The listing builds one solid part. Answer for the finished solid, in the listing's coordinates (mm). A direction names the side the tool comes from. Give positions to 0.01 mm unless a question says otherwise; leave off trailing zeros. Write each loop counter-clockwise with the first axis right and the second up, starting at its lowest first coordinate (ties: lowest second). Pieces come first, ordered by that corner, then holes. Notation, with made-up numbers: M 14,-14 L 60,-14 A17 cw 60,7 Z; hole C 44,-6 d8. An arc over 180 degrees is marked long. Return JSON: item names as keys, results as strings.
from build123d import *
from build123d.topology import SkipClean

# Parameters (mm, degrees)
BOSS_EXTRUDE1_DEPTH      = 41
BOSS_EXTRUDE1_DEPTH_BACK = 18
SKETCH2_R                = 8.000000000000004
SKETCH3_R                = 9.5
BOSS_EXTRUDE2_DEPTH      = 28.5
BOSS_EXTRUDE3_DEPTH      = 5
BOSS_EXTRUDE4_DEPTH      = 25.451834
M3_5_TAPPED_HOLE1_D      = 2.9
FILLET2_R                = 2
SKETCH14_R               = 8.000000000000004
BOSS_EXTRUDE5_DEPTH      = 2
FILLET10_R               = 1
FILLET10_OF_MIRROR2_R    = 1
FILLET11_R               = 1
FILLET12_R               = 2
SKETCH15_W               = 47.04564696040835
SKETCH15_H               = 19.155839546122916
CUT_EXTRUDE2_DEPTH       = 123.75548779255048
SKETCH16_W               = 50.32184914639417
SKETCH16_H               = 9.010919354068848
CUT_EXTRUDE3_DEPTH       = 123.68683594132897


# Some blends are built 0.0001 mm under size
with BuildPart() as part:
    # Sketch2 → Boss-Extrude1 (new, two sides: drawn at the far end of the back side and taken through both)
    with BuildSketch(Plane.XY.offset(-BOSS_EXTRUDE1_DEPTH_BACK)):
        with BuildLine():
            Line((-12.5, -12.500000000000002), (12.5, -12.500000000000002))
            Line((12.5, -12.500000000000002), (12.5, 5.999999999999994))
            Line((12.5, 5.999999999999994), (12.5, 12.951833846988604))
            ThreePointArc((12.5, 12.951833846988604), (9.463639319119588, 15.311418315675832), (5.995365002334926, 16.97220075561143))
            Line((5.995365002334926, 16.97220075561143), (-1.0000000000000027, 16.97220075561143))
            Line((-1.0000000000000027, 16.97220075561143), (-5.995365002334937, 16.972200755611425))
            ThreePointArc((-5.995365002334937, 16.972200755611425), (-9.463639319119597, 15.311418315675827), (-12.5, 12.951833846988608))
            Line((-12.5, 12.951833846988608), (-12.5, 6.000000000000001))
            Line((-12.5, 6.000000000000001), (-12.5, -12.500000000000002))
        make_face()
        Circle(SKETCH2_R, mode=Mode.SUBTRACT)
    extrude(amount=BOSS_EXTRUDE1_DEPTH + BOSS_EXTRUDE1_DEPTH_BACK)

    # Sketch3 → Boss-Extrude2 (add)
    with BuildSketch(Plane.XY.offset(41)):
        with BuildLine():
            Line((-1.0000000000000016, 17.97498435543818), (0.727272727272726, 17.97498435543818))
            Line((0.727272727272726, 17.97498435543818), (8.769260939312526, 17.974984355438174))
            ThreePointArc((8.769260939312526, 17.974984355438174), (11.304195151298408, 16.498944571740374), (13.595959595959597, 14.667988364633844))
            Line((13.595959595959597, 14.667988364633844), (13.595959595959597, 6.224872228225638))
            Line((13.595959595959597, 6.224872228225638), (13.595959595959597, -12.5))
            Line((13.595959595959597, -12.5), (-13.500000000000002, -12.500000000000004))
            Line((-13.500000000000002, -12.500000000000004), (-13.500000000000002, 6.223411383455548))
            Line((-13.500000000000002, 6.223411383455548), (-13.500000000000002, 14.756354563373698))
            ThreePointArc((-13.500000000000002, 14.756354563373698), (-11.250328445445001, 16.535722236104803), (-8.769260939312526, 17.97498435543818))
            Line((-8.769260939312526, 17.97498435543818), (-1.0000000000000016, 17.97498435543818))
        make_face()
        with Locations(Location((-1.73e-15, 0, 0), (0, 0, 180))):
            Circle(SKETCH3_R, mode=Mode.SUBTRACT)
    boss_extrude2 = extrude(amount=BOSS_EXTRUDE2_DEPTH)

    # Mirror1: Boss-Extrude2 across plane
    add(boss_extrude2.mirror(Plane.XY.offset(11.5)))

    # Sketch4 → Boss-Extrude3 (add)
    with BuildSketch(Plane.XZ.offset(12.500000000000002)):
        Polygon((-13.500000000000002, 41), (-13.500000000000002, 69.5), (-18.500000000000004, 69.5), (-18.500000000000004, 42.75), (-18.500000000000004, 36.00000000000001), (-17.5, 36.00000000000001), (-17.5, -13), (-18.500000000000004, -13.000000000000002), (-18.500000000000004, -46.5), (-13.500000000000002, -46.5), (-13.500000000000002, -18.000000000000004), (-12.499999999999998, -18.000000000000004), (-12.5, 41), align=None)
        Polygon((18.595959595959595, 69.5), (13.595959595959597, 69.5), (13.595959595959597, 41), (12.5, 41), (12.5, -18.000000000000004), (13.595959595959597, -18.000000000000004), (13.595959595959597, -46.5), (18.5959595959596, -46.5), (18.595959595959595, -13), (17.5, -13.000000000000002), (17.5, 36.00000000000001), (18.595959595959595, 36.00000000000001), (18.595959595959595, 42.75), align=None)
        Polygon((13.595959595959597, -18.000000000000004), (12.5, -18.000000000000004), (12.5, 41), (13.595959595959597, 41), (13.595959595959597, 69.5), (-13.500000000000002, 69.5), (-13.500000000000002, 41), (-12.5, 41), (-12.499999999999998, -18.000000000000004), (-13.500000000000002, -18.000000000000004), (-13.500000000000002, -46.5), (13.595959595959597, -46.5), align=None)
    extrude(amount=BOSS_EXTRUDE3_DEPTH)

    # Sketch5 → Boss-Extrude4 (add)
    with BuildSketch(Plane(origin=(0, -12.500000000000002, 0), x_dir=(1, 0, 0), z_dir=(0, 1, 0))):
        Polygon((13.595959595959597, -41), (13.595959595959597, -69.5), (18.595959595959595, -69.5), (18.595959595959595, -36.00000000000001), (17.5, -36.00000000000001), (17.5, 13.000000000000002), (18.595959595959595, 13.000000000000002), (18.595959595959595, 46.5), (13.595959595959597, 46.5), (13.595959595959597, 18.000000000000004), (12.5, 18.000000000000004), (12.5, -41), align=None)
        Polygon((-18.500000000000004, -69.5), (-13.500000000000002, -69.5), (-13.500000000000002, -41), (-12.5, -41), (-12.499999999999998, 18.000000000000004), (-13.500000000000002, 18.000000000000004), (-13.500000000000002, 46.5), (-18.5, 46.5), (-18.500000000000004, 13.000000000000002), (-17.5, 13.000000000000002), (-17.5, -36.00000000000001), (-18.500000000000004, -36.00000000000001), align=None)
    extrude(amount=BOSS_EXTRUDE4_DEPTH)

    # M3.5 Tapped Hole1 (through all)
    with Locations(Plane(origin=(-1.179e-14, 16.97220075561143, 0), x_dir=(1, 6.9e-16, 0), z_dir=(-6.9e-16, 1, 0))):
        with Locations((-12.5, 15), (12.5, 15), (12.5, 35), (-12.5, 35)):
            m3_5_tapped_hole1 = Hole(M3_5_TAPPED_HOLE1_D / 2)

    # Fillet2
    fillet2_edges = [part.edges().sort_by_distance(p)[0] for p in [
        (18.595959595959595, 12.951834, -29.75),
        (-18.5, 12.951834, -29.75),
    ]]
    fillet(fillet2_edges, radius=FILLET2_R - 0.0001)  # a hair under: the kernel refuses the full size

    # Sketch14 → Boss-Extrude5 (add)
    with SkipClean():  # the faces are left unmerged after this step: merging them gives an invalid solid
        with BuildSketch(Plane.XY.offset(69.5)):
            with BuildLine():
                Line((13.595959595959597, 12.951833846988603), (-13.500000000000002, 12.951833846988603))
                Line((-13.500000000000002, 12.951833846988603), (-16.5, 12.951833846988603))
                ThreePointArc((-16.5, 12.951833846988604), (-17.914213562373096, 12.366047409361698), (-18.5, 10.951833846988603))
                Line((-18.500000000000004, 10.951833846988603), (-18.500000000000004, -17.5))
                Line((-18.500000000000004, -17.5), (18.595959595959595, -17.5))
                Line((18.595959595959595, -17.5), (18.595959595959595, 10.951833846988603))
                ThreePointArc((18.595959595959595, 10.951833846988603), (18.01017315833269, 12.366047409361698), (16.595959595959595, 12.951833846988603))
                Line((16.595959595959595, 12.951833846988604), (13.595959595959597, 12.951833846988603))
            make_face()
            Circle(SKETCH14_R, mode=Mode.SUBTRACT)
        boss_extrude5 = extrude(amount=BOSS_EXTRUDE5_DEPTH)

    # Fillet10
    fillet10_edges = [part.edges().sort_by_distance(p)[0] for p in [
        (0.04797979797979934, 12.951833846988603, 71.5),
        (-8.000000000000004, 9.8e-16, 71.5),
        (-17.914213562373096, 12.366047409361698, 71.5),
        (-18.500000000000004, -3.2740830765056987, 71.5),
        (0.04797979797979579, -17.5, 71.5),
        (18.595959595959595, -3.2740830765056987, 71.5),
        (18.01017315833269, 12.366047409361698, 71.5),
    ]]
    fillet(fillet10_edges, radius=FILLET10_R)

    # Mirror2: Boss-Extrude5 across plane
    with SkipClean():  # the faces are left unmerged after this step: merging them gives an invalid solid
        add(boss_extrude5.mirror(Plane.XY.offset(11.5)))

    # Fillet10 of Mirror2
    fillet10_of_mirror2_edges = [part.edges().sort_by_distance(p)[0] for p in [
        (0.04797979797979934, 12.951833846988603, -48.5),
        (-8.000000000000004, 9.8e-16, -48.5),
        (-17.914213562373096, 12.366047409361698, -48.5),
        (-18.500000000000004, -3.2740830765056987, -48.5),
        (0.04797979797979579, -17.5, -48.5),
        (18.595959595959595, -3.2740830765056987, -48.5),
        (18.01017315833269, 12.366047409361698, -48.5),
    ]]
    fillet(fillet10_of_mirror2_edges, radius=FILLET10_OF_MIRROR2_R)

    # Fillet11
    fillet11_edges = [part.edges().sort_by_distance(p)[0] for p in [
        (11.304195151298412, 16.498944571740378, 69.5),
        (1.78e-15, 17.974984355438178, 69.5),
        (-11.250328445445, 16.535722236104803, 69.5),
        (-11.250328445445, 16.535722236104803, -46.5),
        (1.78e-15, 17.974984355438178, -46.5),
        (11.304195151298412, 16.498944571740378, -46.5),
    ]]
    fillet(fillet11_edges, radius=FILLET11_R)

    # Fillet12
    # the kernel refuses this fillet: 2 mm, written as the material it adds along each edge
    with BuildSketch(Plane(origin=(-1.73e-15, 0, 41), x_dir=(-1, 1.2e-16, 0), z_dir=(1.2e-16, 1, 0))) as fillet12_piece_1:
        with BuildLine():
            CenterArc((7.5, 1.9364916731037098), FILLET12_R, 284.47751218593, 75.52248781407002)
            Line((8.000000000000004, 0), (8.010000000000003, -0.03872983346207093))
            ThreePointArc((8.010000000000003, -0.03872983346207093), (8.750000000000002, -0.03999999999999915), (9.5, -0.03999999999999915))
            Line((9.5, -0.03999999999999915), (9.54, 0))
            Line((9.54, 0), (9.54, 1.9364916731037098))
            Line((9.54, 1.9364916731037098), (9.5, 1.9364916731037098))
        make_face()
    revolve(axis=Axis((-1.73e-15, 0, 41), (0, 0, 1)))
    # the kernel refuses this fillet: 2 mm, written as the material it takes off along each edge
    with BuildSketch(Plane(origin=(-1.73e-15, 0, -18), x_dir=(1, 0, 0), z_dir=(0, -1, 0))) as fillet12_2_piece_1:
        with BuildLine():
            CenterArc((10.000000000000004, 1.9364916731037063), FILLET12_R, 180, 75.52248781406996)
            Line((8.000000000000004, 1.9364916731037063), (7.9600000000000035, 1.9364916731037063))
            Line((7.9600000000000035, 1.9364916731037063), (7.9600000000000035, 0))
            Line((7.9600000000000035, 0), (8.000000000000004, -0.03999999999999915))
            ThreePointArc((8.000000000000004, -0.03999999999999915), (8.750000000000002, -0.03999999999999915), (9.49, -0.03872983346207448))
            Line((9.49, -0.03872983346207448), (9.5, 0))
        make_face()
    revolve(axis=Axis((-1.73e-15, 0, -18), (0, 0, 1)), mode=Mode.SUBTRACT)

    # Mirror3: M3.5 Tapped Hole1 across plane
    with SkipClean():  # the faces are left unmerged after this step: merging them gives an invalid solid
        add(m3_5_tapped_hole1.mirror(Plane.XY.offset(11.5)), mode=Mode.SUBTRACT)

    # Sketch15 → Cut-Extrude2 (cut, through all)
    with BuildSketch(Plane.XY.offset(71.50000000000001)):
        with Locations((2.6415149640881275, 9.577919773061458)):
            Rectangle(SKETCH15_W, SKETCH15_H)
    extrude(amount=-CUT_EXTRUDE2_DEPTH, mode=Mode.SUBTRACT)

    # Sketch16 → Cut-Extrude3 (cut, through all)
    with BuildSketch(Plane(origin=(0, 0, -48.50000000000001), x_dir=(-1, 0, 0), z_dir=(0, 0, -1))):
        with Locations((0.38733031574332877, -17.005459677034427)):
            Rectangle(SKETCH16_W, SKETCH16_H)
    extrude(amount=-CUT_EXTRUDE3_DEPTH, mode=Mode.SUBTRACT)


solid = part.part
Item 1: Which of the six approach directions +Z, -Z, +X, -X, +Y, -Y give full straight-line access (tool end or side, diameter ignored) to faces 1 (the cylindrical face through (12.814, -6.337, -33.584)), 2 (the flat face through (-17.5, -6, 12)), 3 (the flat face through (-1.5, -8.2, 69.5))?
Geometry results:
{"face 1": "+Y, -Y", "face 2": "-X, +Y, -Y", "face 3": "+Y"}
Item 2: Determine the mould class of faces 4 (the cylindrical face through (0, -8, 70)), 5 (the flat face through (17.5, -6, 12)), 6 (the flat face through (0, -10, -48.5)), 7 (the flat face through (-18.5, -6, -30)) for opening direction X: +X half, -X half, draft (parallel to the pull), parting line (faces both ways), or undercut.
Geometry results:
{"face 4": "undercut", "face 5": "+X half", "face 6": "draft", "face 7": "-X half"}
Item 3: Given pin 1 Ø4.5 at (x, z) = (-12.5, 38) entering from +Y; pin 2 Ø3 at (x, y) = (4.5, -5) entering from +Z; pin 3 Ø4 at (y, z) = (-8, 11.5) entering from +X; pin 4 Ø1.2 at (x, y) = (18.5, -3.5) entering from +Z, each flat-ended and moving along its own axis, determine where each tip first touches the part or whether it passes through.
Geometry results:
{"pin 1": "stops at y = 0", "pin 2": "stops at z = 71.13", "pin 3": "stops at x = 17.5", "pin 4": "stops at z = 71.45"}
Item 4: A cutting plane is placed at D-D, the plane y = -2. Count the separate pieces of the cut face and the enclosed holes in it, plus the area to 3 significant figures.
Geometry results:
{"separate pieces": "2", "enclosed holes": "8", "area": "2,260 mm2"}
Item 5: A cutting plane is placed at B-B, the plane z = 58. Write down the section's boundary in (x, y), plus the area to 3 significant figures.
Geometry results:
{"outline": "M -18.5,-12.5 L -13.95,-12.5 L -13.95,0 L -18.5,0 Z; M -11.05,-12.5 L 11.05,-12.5 L 11.05,0 L 9.5,0 A9.5 cw -9.5,0 L -11.05,0 Z; M 13.95,-12.5 L 18.6,-12.5 L 18.6,0 L 13.95,0 Z", "area": "249 mm2"}
Item 6: A cutting plane is placed at A-A, the plane x = 12.5. Write down the section's boundary in (y, z), plus the area to 4 significant figures.
Geometry results:
{"outline": "M -12.5,-48.5 L 0,-48.5 L 0,-36.45 L -12.5,-36.45 Z; M -12.5,-33.55 L 0,-33.55 L 0,-16.45 L -12.5,-16.45 Z; M -12.5,-13.55 L 0,-13.55 L 0,36.55 L -12.5,36.55 Z; M -12.5,39.45 L 0,39.45 L 0,56.55 L -12.5,56.55 Z; M -12.5,59.45 L 0,59.45 L 0,71.5 L -12.5,71.5 Z", "area": "1,355 mm2"}
Item 7: Find the intervals of material crossed by line 1 (Z direction, x = -12.5, y = -8); line 2 (X direction, y = -9, z = 38); line 3 (X direction, y = -10.25, z = -36), in increasing order.
Geometry results:
{"line 1": "z = -48.5 to -36.45, -33.55 to -16.45, -13.55 to 36.55, 39.45 to 56.55, 59.45 to 71.5", "line 2": "x = -18.5 to -13.95, -11.05 to 11.05, 13.95 to 18.6", "line 3": "x = -18.5 to -13.55, -11.45 to 11.45, 13.55 to 18.6"}
Item 8: A cutting plane is placed at C-C, the plane z = -23. Write down the section's boundary in (x, y), plus the area to 3 significant figures.
Geometry results:
{"outline": "M -18.5,-12.5 L 18.6,-12.5 L 18.6,0 L 9.5,0 A9.5 cw -9.5,0 L -18.5,0 Z", "area": "322 mm2"}
